Could you check a few things on this model? Use its own coordinates, in mm. A direction names the side the tool comes from. Coordinates: 2 decimals unless noted, no trailing zeros. Order: outer loops, then holes, each group sorted by start corner. A loop starts at its lowest first (then second) coordinate and runs counter-clockwise, first axis right, second up. Notation, with made-up numbers: M 33.25,12.25 L 65.25,12.25 A26 ccw 65.25,30.25 Z; hole C -37,-21.5 d9. An arc over 180 degrees is marked long. One line per question, with ' | ' between items. Start each with the question number.
from build123d import *

# Parameters (mm, degrees)
M3_CLEARANCE_HOLE1_D = 3.4
CIRPATTERN1_COUNT    = 4
BOSS_EXTRUDE1_START  = -6.876
BOSS_EXTRUDE1_DEPTH  = 6.876
CHAMFER1_SIZE        = 0.75
CHAMFER2_SIZE        = 1


with BuildPart() as part:
    # Sketch1 → Revolve1 (revolve)
    with BuildSketch(Plane.XY, mode=Mode.PRIVATE) as revolve1_sk:
        Polygon((6.8, 0), (6.8, 4.953), (5.2, 4.953), (5.2, 11.829), (7.112, 11.829), (8.9, 10.1665), (8.9, 7.1665), (23, 7.1665), (23, 0), align=None)
    revolve(revolve1_sk.sketch.rotate(Axis((0, 0, 0), (0, 1, 0)), 90), axis=Axis((0, 0, 0), (0, 1, 0)))

    # M3 Clearance Hole1 (through all)
    with Locations(Plane.XZ):
        with Locations((-20, 0)):
            m3_clearance_hole1 = Hole(M3_CLEARANCE_HOLE1_D / 2)

    # CirPattern1: M3 Clearance Hole1 ×4 about axis
    cirpattern1_axis = Axis((0, 0, 0), (0, 1, 0))
    for i in range(1, CIRPATTERN1_COUNT):
        add(m3_clearance_hole1.rotate(cirpattern1_axis, i * 360 / CIRPATTERN1_COUNT), mode=Mode.SUBTRACT)

    # Sketch4 → Boss-Extrude1 (add)
    with BuildSketch(Plane.XZ.offset(-4.953).offset(BOSS_EXTRUDE1_START)):
        with BuildLine():
            Line((0.700412138, 5.152613205), (4.112087862, 3.182881307))
            ThreePointArc((4.112087862, 3.182881307), (2.6, 4.5033321), (0.700412138, 5.152613205))
        make_face()
        with BuildLine():
            ThreePointArc((4.8125, -1.969731898), (5.2, 0), (4.8125, 1.969731898))
            Line((4.8125, 1.969731898), (4.8125, -1.969731898))
        make_face()
        with BuildLine():
            Line((-4.112087862, 3.182881307), (-0.700412138, 5.152613205))
            ThreePointArc((-0.700412138, 5.152613205), (-2.6, 4.5033321), (-4.112087862, 3.182881307))
        make_face()
        with BuildLine():
            ThreePointArc((0.700412138, -5.152613205), (2.6, -4.5033321), (4.112087862, -3.182881307))
            Line((4.112087862, -3.182881307), (0.700412138, -5.152613205))
        make_face()
        with BuildLine():
            Line((-4.8125, -1.969731898), (-4.8125, 1.969731898))
            ThreePointArc((-4.8125, 1.969731898), (-5.2, 0), (-4.8125, -1.969731898))
        make_face()
        with BuildLine():
            ThreePointArc((-4.112087862, -3.182881307), (-2.6, -4.5033321), (-0.700412138, -5.152613205))
            Line((-0.700412138, -5.152613205), (-4.112087862, -3.182881307))
        make_face()
    extrude(amount=BOSS_EXTRUDE1_DEPTH)

    # Chamfer1
    chamfer1_edges = [part.edges().sort_by_distance(p)[0] for p in [
        (0, 0, 6.8),
    ]]
    chamfer(chamfer1_edges, length=CHAMFER1_SIZE)

    # Chamfer2
    chamfer2_edges = [part.edges().sort_by_distance(p)[0] for p in [
        (0, 7.1665, 23),
    ]]
    chamfer(chamfer2_edges, length=CHAMFER2_SIZE)


solid = part.part
(1) Imagine slicing it at A-A, the plane z = 0. Count the separate pieces of the cut face and the enclosed holes in it, plus the area to 3 significant figures.
(2) On a 3-axis mill with a long thin cutter (end or side, diameter ignored), from which of +Z, -Z, +X, -X, +Y, -Y can I reach the whole of each face in a straight line? I mean faces 4 (the flat face through (-2.382, 8.439, -4.182)), 5 (the cylindrical face through (6.64, 2.88, 1.47)), 6 (the conical face through (6.409, 11.725, -3.333)). Say none if no direction works.
(3) For P1, Ø1, axis at y = 7.5, z = 16.5, coming from the +X side; P2, Ø1.5, axis at y = 6, z = -18, coming from the +X side; P3, Ø3, axis at y = 7.5, z = 1, coming from the +X side, each with a flat end and sliding along its axis, tell me the tip position at first contact or that it passes through.
(4) We'd pull the mould along X, two halves only. Please class faces 1 (the flat face through (4.812, 8, 0)), 2 (the flat face through (0, 0, -10)), 3 (the cylindrical face through (-22.804, 3.04, 2.994)): +X half, -X half, draft (parallel to the pull), parting line (faces both ways), or undercut.
(5) Imagine slicing it at B-B, the plane y = 8. Write out the boundary of the cut face in (x, z), plus the area to 3 significant figures.
(6) If I drill on line 1 along Y through (x, z) = (10.5, 14.5); line 2 along X through (y, z) = (4.75, 20); line 3 along Z through (x, y) = (-3.5, 9), over which ranges is the centre line in solid material (lowest first)? Write a range as from..to.
(7) Imagine slicing it at D-D, the plane y = 2.5. Write out the boundary of the cut face in (x, z).
Answers:
1) separate pieces: 4 | enclosed holes: 0 | area: 226 mm²
2) face 4: +Y, -Y | face 5: -Y | face 6: +Y
3) P1: x = 14.98 | P2: x = 15.21 | P3: x = 23
4) face 1: undercut | face 2: draft | face 3: parting line
5) outline: C 0,0 d17.8; hole M -4.81,-1.97 A5.2 ccw -4.11,-3.18 L -0.7,-5.15 A5.2 ccw 0.7,-5.15 L 4.11,-3.18 A5.2 ccw 4.81,-1.97 L 4.81,1.97 A5.2 ccw 4.11,3.18 L 0.7,5.15 A5.2 ccw -0.7,5.15 L -4.11,3.18 A5.2 ccw -4.81,1.97 Z | area: 170 mm²
6) line 1: 0..7.17 | line 2: -11.36..-1.7, 1.7..11.36 | line 3: -8.18..-3.54, 3.54..8.18
7) outline: C 0,0 d46; hole C -20,0 d3.4; hole C 0,0 d13.6; hole C 0,-20 d3.4; hole C 0,20 d3.4; hole C 20,0 d3.4
